from build123d import *

# Parameters (mm, degrees)
SKETCH1_R               = 10
SKETCH1_R_2             = 5
BOSS_EXTRUDE1_DEPTH     = 10
CHAMFER1_SIZE           = 0.5
CUT_EXTRUDE1_REACH      = 19.321
CUT_EXTRUDE1_END_RADIUS = 10
SKETCH19_R              = 2.5


with BuildPart() as part:
    # Sketch1 → Boss-Extrude1 (new body)
    with BuildSketch(Plane(origin=(0, 0, 0), x_dir=(1, 0, 0), z_dir=(0, 1, 0))):
        with Locations(Location((0, 0, 0), (0, 0, 270))):
            Circle(SKETCH1_R)
        with Locations(Location((0, 0, 0), (0, 0, 270))):
            Circle(SKETCH1_R_2, mode=Mode.SUBTRACT)
    extrude(amount=BOSS_EXTRUDE1_DEPTH)

    # Chamfer1
    chamfer1_edges = [part.edges().sort_by_distance(p)[0] for p in [
        (0, 10, -10),
    ]]
    chamfer(chamfer1_edges, length=CHAMFER1_SIZE)

    # Cut-Extrude1: up to this cylinder (the profile starts inside it)
    cut_extrude1_end = Plane(origin=(0, 5, 0), z_dir=(0, -1, 0)) * Cylinder(CUT_EXTRUDE1_END_RADIUS, 59.642, mode=Mode.PRIVATE)
    # Sketch19 → Cut-Extrude1 (cut, up to the surface)
    with BuildSketch(Plane(origin=(0, 0, 0), x_dir=(0, 0, -1), z_dir=(1, 0, 0)), mode=Mode.PRIVATE) as cut_extrude1_sk1:
        with Locations((0, 5)):
            Circle(SKETCH19_R)
    cut_extrude1_tool1 = extrude(cut_extrude1_sk1.sketch, amount=-CUT_EXTRUDE1_REACH, mode=Mode.PRIVATE) & cut_extrude1_end
    add(cut_extrude1_tool1.solids().sort_by_distance((0, 5, 0))[0], mode=Mode.SUBTRACT)


solid = part.part
Geometry: final body of the model. Coordinates: model frame, mm. Give positions to 0.01 mm unless a question says otherwise; leave off trailing zeros. Order: outer loops, then holes, each group sorted by start corner. A loop starts at its lowest first (then second) coordinate and runs counter-clockwise, first axis right, second up. Notation, with made-up numbers: (30.25, 64) -> (61.25, 64) arc R7 cw to (61.25, 72) -> close; hole circle Ø10 at (18.5, 71.25). An arc over 180 degrees is marked (long way). Answer as a JSON object with one key per item and string values.
Q1. First-contact query: pin 1 (4 mm diameter, centred on y = 8.5, z = -7.5, fed in from -X); pin 2 (3 mm diameter, centred on x = 3.5, y = 4, fed in from +Z); pin 3 (4 mm diameter, centred on y = 4, z = -5, fed in from +X); pin 4 (12 mm diameter, centred on x = 7, z = 1.5, fed in from -Y). Flat tips, straight axial feed; report the tip coordinate or a pass-through.
Entries:
{"pin 1": "stops at x = -8.35", "pin 2": "stops at z = 9.8", "pin 3": "stops at x = 9.54", "pin 4": "stops at y = 0"}
Q2. Section B-B (x = 0). Output: boundary loops of the cut face in (y, z), plus the area to 4 significant figures.
Entries:
{"outline": "(0, -10) -> (9.5, -10) -> (10, -9.5) -> (10, -5) -> (0, -5) -> close; (0, 5) -> (10, 5) -> (10, 9.5) -> (9.5, 10) -> (0, 10) -> close", "area": "99.75 mm^2"}
Q3. Section A-A (z = 0). Output: boundary loops of the cut face in (x, y).
Entries:
{"outline": "(-10, 0) -> (-5, 0) -> (-5, 2.5) -> (-10, 2.5) -> close; (-10, 7.5) -> (-5, 7.5) -> (-5, 10) -> (-9.5, 10) -> (-10, 9.5) -> close; (5, 0) -> (10, 0) -> (10, 9.5) -> (9.5, 10) -> (5, 10) -> close"}
Q4. Section C-C (y = 1). Output: boundary loops of the cut face in (x, z), plus the area to 3 significant figures.
Entries:
{"outline": "circle Ø20 at (0, 0); hole circle Ø10 at (0, 0)", "area": "236 mm^2"}
Q5. Material intervals for probe 1 along Y at (x, z) = (-7.5, 0); probe 2 along X at (y, z) = (4, 0); probe 3 along X at (y, z) = (8.75, -0.5), sorted ascending.
Entries:
{"probe 1": "y = 0 to 2.5, 7.5 to 10", "probe 2": "x = 5 to 10", "probe 3": "x = -9.99 to -4.97, 4.97 to 9.99"}
Q6. Section D-D (y = 5). Output: boundary loops of the cut face in (x, z), plus the area to 3 significant figures.
Entries:
{"outline": "(-9.68, -2.5) arc R10 ccw (long way) to (-9.68, 2.5) -> (-4.33, 2.5) arc R5 cw (long way) to (-4.33, -2.5) -> close", "area": "210 mm^2"}
Q7. Draft query along Y for faces 1 (the cylindrical face through (-7.13, 2.56, 0.54)), 2 (the flat face through (5, 0, 2)), 3 (the flat face through (-4, 10, 4)). Return one class per face: released by +Y, released by -Y, zero draft, split by the parting line, or undercut.
Entries:
{"face 1": "undercut", "face 2": "released by -Y", "face 3": "released by +Y"}
